The model under review builds one solid part; all positions refer to its coordinate system, in mm. Give positions to 0.01 mm unless a question says otherwise; leave off trailing zeros. Order: outer loops, then holes, each group sorted by start corner. A loop starts at its lowest first (then second) coordinate and runs counter-clockwise, first axis right, second up.
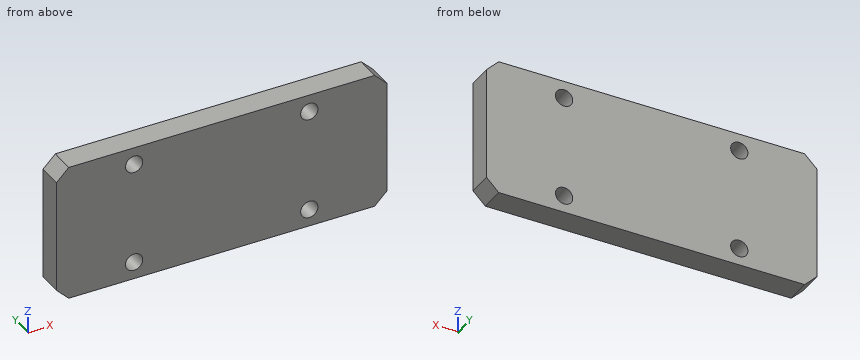
```python
from build123d import *

# Parameters (mm, degrees)
BOSS_EXTRUDE1_DEPTH = 56
SKETCH3_R           = 3.5
CUT_EXTRUDE1_DEPTH  = 10
CHAMFER1_SIZE       = 5


with BuildPart() as part:
    # Sketch2 → Boss-Extrude1 (new body)
    with BuildSketch(Plane.XY):
        Polygon((46, 10), (-46, 10), (-67, 10), (-67, 0), (-45, 0), (45, 0), (67, 0), (67, 10), align=None)
    extrude(amount=BOSS_EXTRUDE1_DEPTH)

    # Sketch3 → Cut-Extrude1 (cut)
    with BuildSketch(Plane(origin=(0, 10, 0), x_dir=(1, 0, 0), z_dir=(0, 1, 0))):
        with Locations(Location((-35.5, -7.055, 0), (0, 0, 180))):
            Circle(SKETCH3_R)
        with Locations(Location((35.5, -7.055, 0), (0, 0, 180))):
            Circle(SKETCH3_R)
        with Locations(Location((-35.5, -48.945, 0), (0, 0, 180))):
            Circle(SKETCH3_R)
        with Locations(Location((35.5, -48.945, 0), (0, 0, 180))):
            Circle(SKETCH3_R)
    extrude(amount=-CUT_EXTRUDE1_DEPTH, mode=Mode.SUBTRACT)

    # Chamfer1
    chamfer1_edges = [part.edges().sort_by_distance(p)[0] for p in [
        (67, 5, 0),
        (-67, 5, 56),
        (67, 5, 56),
        (-67, 5, 0),
    ]]
    chamfer(chamfer1_edges, length=CHAMFER1_SIZE)


solid = part.part
```
1. Take a section at B-B (y = 8.5). Write out the cut boundary in (x, z) (3 decimals), and give its area (3 significant figures).
2. Take a section at A-A (x = 35.5). Write out the cut boundary in (y, z) (3 decimals).
3. To check wall thickness, follow line 1 (Z direction, x = -35.5, y = 9.5) (3 decimals); line 2 (X direction, y = 5.75, z = 50.5); line 3 (X direction, y = 9.25, z = 5). State the ranges of each line that lie inside material, in increasing order.
4. Insertion check: pin 1 (9 mm diameter, centred on x = -35.5, z = 48.945, fed in from -Y). The pin has a flat end and moves straight along its axis. Give the tip position at first contact, or say it passes through.
Answer:
1. outline: (-67, 5) - (-62, 0) - (62, 0) - (67, 5) - (67, 51) - (62, 56) - (-62, 56) - (-67, 51) - close; hole circle Ø7 at (-35.5, 7.055); hole circle Ø7 at (-35.5, 48.945); hole circle Ø7 at (35.5, 7.055); hole circle Ø7 at (35.5, 48.945)
1. area: 7,300 mm2
2. outline: (0, 0) - (10, 0) - (10, 3.555) - (0, 3.555) - close; (0, 10.555) - (10, 10.555) - (10, 45.445) - (0, 45.445) - close; (0, 52.445) - (10, 52.445) - (10, 56) - (0, 56) - close
3. line 1: z = 0 to 3.555, 10.555 to 45.445, 52.445 to 56
3. line 2: x = -67 to -38.64, -32.36 to 32.36, 38.64 to 67
3. line 3: x = -67 to -38.33, -32.67 to 32.67, 38.33 to 67
4. pin 1: stops at y = 0
